```python
from build123d import *

# Parameters (mm, degrees)
F0_R     = 2.54
F1_DEPTH = 1.27
F3_DEPTH = 1.778
F4_R     = 1.4097
F5_DEPTH = 17.78
F6_R     = 1.27


with BuildPart() as f1:
    # F0 (on Right) → F1 (new body)
    with BuildSketch(Plane.YZ):
        Circle(F0_R)
    extrude(amount=F1_DEPTH)

    # F2 (on face) → F3 (join)
    with BuildSketch(Plane(origin=(0, 0, 0), x_dir=(0, -1, 0), z_dir=(-1, 0, 0))):
        Polygon((-2.0598, -1.369699), (0.156294, -2.468689), (2.216094, -1.09899), (2.0598, 1.369699), (-0.156294, 2.468689), (-2.216094, 1.09899), align=None)
        Polygon((1.805483, -0.893684), (0.128788, -2.010436), (-1.676694, -1.116752), (-1.805483, 0.893684), (-0.128788, 2.010436), (1.676694, 1.116752), align=None, mode=Mode.SUBTRACT)
    extrude(amount=F3_DEPTH)

    # F4 (on face) → F5 (join)
    with BuildSketch(Plane.YZ.offset(1.27)):
        Circle(F4_R)
    extrude(amount=F5_DEPTH)

    # F6
    f6_edges = [f1.edges().sort_by_distance(p)[0] for p in [
        (19.05, -1.4097, 0),
    ]]
    fillet(f6_edges, radius=F6_R)


solid = f1.part
```
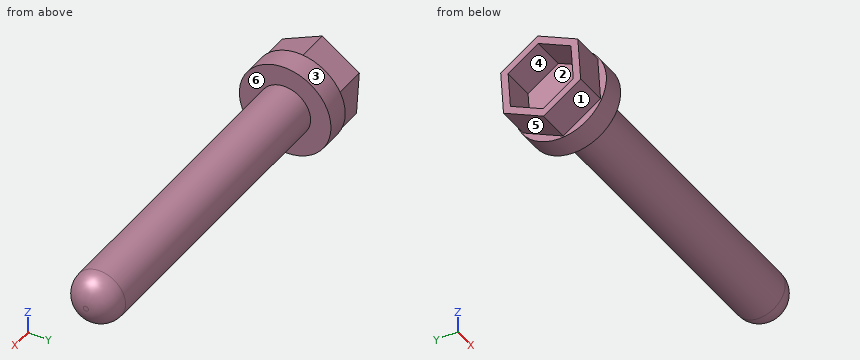
Source: CAD feature listing. Evaluate the final solid. Frame: model axes, mm. Face numbers are marked on the shaded views. A direction names the side the tool comes from. Coordinates: 2 decimals unless noted, no trailing zeros. Loops run counter-clockwise (first coordinate to the right, second up) from the corner with the lowest first, then second, coordinate; pieces in that order, holes last. Notation, with made-up numbers: M -12,56.5 L -2,56.5 A27 ccw -2,90.5 Z; hole C 1,-10 d3. An arc over 180 degrees is marked long. Use a Markdown table: item, result. Add a question column.
Q1. Section query A-A, the plane x = -0.25. Return loops of the section in (y, z), and give its area (3 significant figures).
Q2. Access query for the marked faces 4, 5 and 6. Directions: +Z, -Z, +X, -X, +Y, -Y. A direction counts if a zero-diameter tool reaches every point of the face in a straight line with its end or side. Return the directions, or none.
Q3. Draft query along Y for the marked faces 1, 2 and 3. Return one class per face: pulls with the +Y half, pulls with the -Y half, needs draft (parallel to the pull), parting line crosses it, or undercut.
Q4. Material intervals for L1, parallel to X at y = 1.45, z = 0.8; L2, parallel to Y at x = 5.5, z = 0.05; L3, parallel to X at y = -2, z = 0.05, sorted ascending.
Q5. Section query B-B, the plane x = 2. Return loops of the section in (y, z), and give its area (3 significant figures).
Q6. First-contact query: pin 1 (3 mm diameter, centred on y = -0.5, z = -0.5, fed in from -X); pin 2 (3 mm diameter, centred on x = 12, y = 1, fed in from +Z). Flat tips, straight axial feed; report the tip coordinate or a pass-through.
Result:
| question | item | result |
|---|---|---|
| 1 | outline | M -2.22,-1.1 L -0.16,-2.47 L 2.06,-1.37 L 2.22,1.1 L 0.16,2.47 L -2.06,1.37 Z; hole M -1.81,-0.89 L -0.13,-2.01 L 1.68,-1.12 L 1.81,0.89 L 0.13,2.01 L -1.68,1.12 Z |
| 1 | area | 5.35 mm2 |
| 2 | face 4 | -X |
| 2 | face 5 | -Z, -X, +Y |
| 2 | face 6 | +X |
| 3 | face 1 | pulls with the -Y half |
| 3 | face 2 | undercut |
| 3 | face 3 | parting line crosses it |
| 4 | L1 | x = 0 to 1.27 |
| 4 | L2 | y = -1.41 to 1.41 |
| 4 | L3 | x = -1.78 to 1.27 |
| 5 | outline | C 0,0 d2.82 |
| 5 | area | 6.24 mm2 |
| 6 | pin 1 | stops at x = -1.78 |
| 6 | pin 2 | stops at z = 1.41 |
